Geometry check sheet. Reference: drawing and pictorial views, mm from the part's lowest x, y, z. Coordinates: 2 decimals unless noted, no trailing zeros. Loops run counter-clockwise (first coordinate to the right, second up) from the corner with the lowest first, then second, coordinate; pieces in that order, holes last.
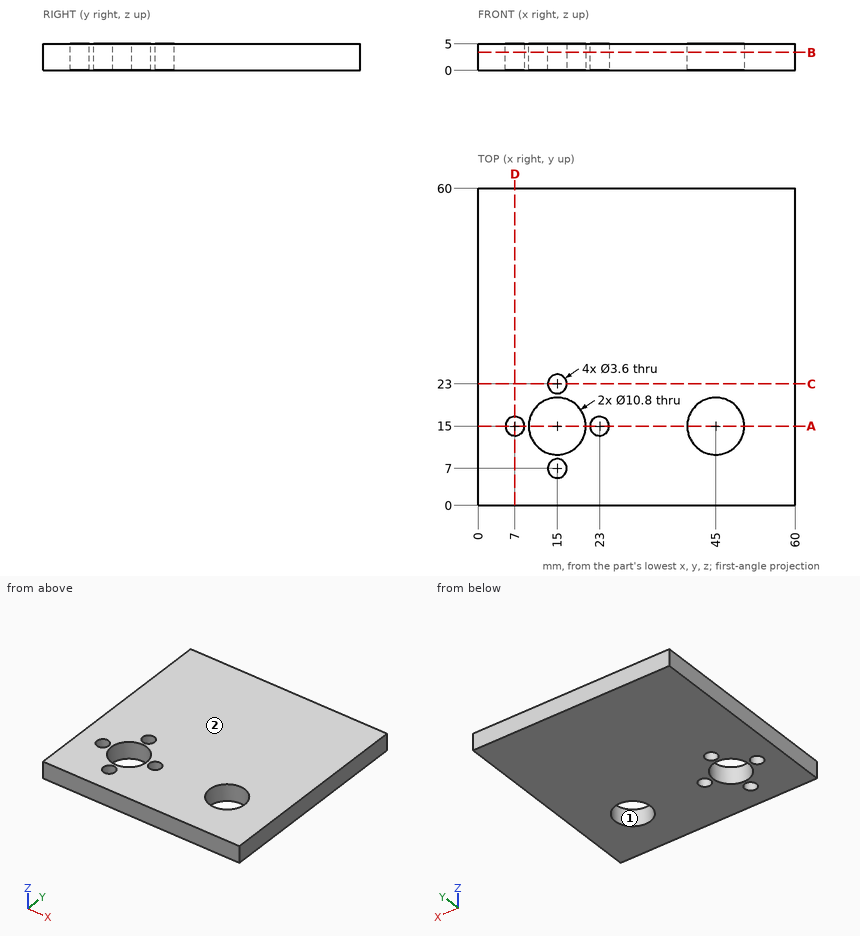
1) Section check B-B on z = 3.4. Record the cut outline in (x, y), and give its area (3 significant figures).
Data:
outline: (0, 0) - (60, 0) - (60, 60) - (0, 60) - close; hole circle Ø3.6 at (7, 15); hole circle Ø10.8 at (15, 15); hole circle Ø3.6 at (15, 7); hole circle Ø3.6 at (15, 23); hole circle Ø3.6 at (23, 15); hole circle Ø10.8 at (45, 15)
area: 3,380 mm2
2) Section check C-C on y = 23. Record the cut outline in (x, z), and give its area (3 significant figures).
Data:
outline: (0, 0) - (13.2, 0) - (13.2, 5) - (0, 5) - close; (16.8, 0) - (60, 0) - (60, 5) - (16.8, 5) - close
area: 282 mm2
3) Depth check by flat-ended pin: pin 1 (2 mm diameter, centred on x = 15, y = 23, fed in from -Z); pin 2 (17.5 mm diameter, centred on x = 45, y = 15, fed in from +Z). Enter the tip coordinate at first touch or a pass-through.
Data:
pin 1: passes through
pin 2: stops at z = 5
4) Section check A-A on y = 15. Record the cut outline in (x, z), and give its area (3 significant figures).
Data:
outline: (0, 0) - (5.2, 0) - (5.2, 5) - (0, 5) - close; (8.8, 0) - (9.6, 0) - (9.6, 5) - (8.8, 5) - close; (20.4, 0) - (21.2, 0) - (21.2, 5) - (20.4, 5) - close; (24.8, 0) - (39.6, 0) - (39.6, 5) - (24.8, 5) - close; (50.4, 0) - (60, 0) - (60, 5) - (50.4, 5) - close
area: 156 mm2
5) Material ranges on probe 1 along Y at (x, z) = (15, 3); probe 2 along Y at (x, z) = (45, 3); probe 3 along Y at (x, z) = (7, 1.3), recorded low to high.
Data:
probe 1: y = 0 to 5.2, 8.8 to 9.6, 20.4 to 21.2, 24.8 to 60
probe 2: y = 0 to 9.6, 20.4 to 60
probe 3: y = 0 to 13.2, 16.8 to 60
6) Mould release check, pull along Y, two halves, no side actions. Record for the marked faces 1 and 2: +Y half, -Y half, draft (parallel to the pull), parting line (faces both ways), or undercut.
Data:
face 1: undercut
face 2: draft
